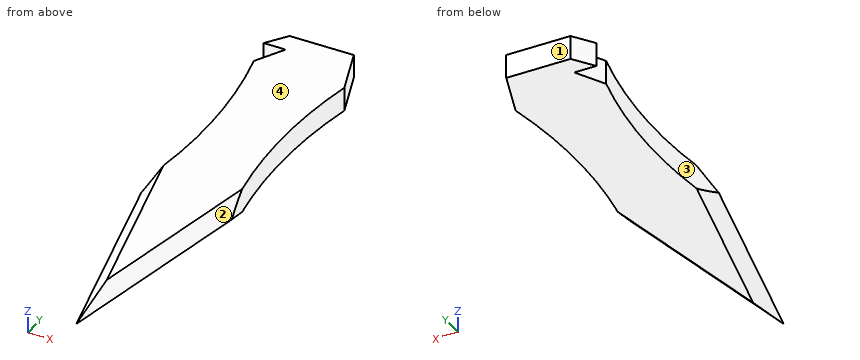
```python
from build123d import *

# Parameters (mm, degrees)
F1_DEPTH = 6.35
F3_DEPTH = 25.4
F5_DEPTH = 6.35
F6_SIZE  = 3.17499


# Not quite as in the source:
# - a fillet or chamfer is up to 0.001 mm smaller than in the source, because OpenCascade refuses the exact size


with BuildPart() as f1:
    # F0 (on Top) → F1 (new body)
    with BuildSketch(Plane.XY):
        Polygon((-21.1028610796, 36.5512275749), (-11.7370359251, 20.3291425525), (0, 29.516665265), (11.7370359251, 20.3291425525), (33.4666037048, 57.9658579735), (26.5181194991, 63.6764243245), (35.1014384706, 60.7974748498), (47.9729409095, 83.0915710438), (43.2239025831, 86.8056491017), (49.1863254635, 85.1932147405), (60.325, 104.4859649666), (44.45, 109.9852262806), (0, 63.5), (-44.45, 109.9852262806), (-60.325, 104.4859649666), (-49.1863254635, 85.1932147405), (-43.2239025831, 86.8056491017), (-47.9729409095, 83.0915710438), (-35.1014384706, 60.7974748498), (-26.5181194991, 63.6764243245), (-33.4666037048, 57.9658579735), align=None)
    extrude(amount=F1_DEPTH)

    # F2 (on face) → F3 (cut)
    with BuildSketch(Plane(origin=(0, 0, 0), x_dir=(1, 0, 0), z_dir=(0, 0, -1))):
        with BuildLine():
            ThreePointArc((-11.7370359251, -75.7744380392), (-8.6743378245, -48.0517902958), (-11.7370359251, -20.3291425525))
            Line((-11.7370359251, -20.3291425525), (-33.4666037048, -57.9658579735))
            Line((-33.4666037048, -57.9658579735), (-26.5181194991, -63.6764243245))
            Line((-26.5181194991, -63.6764243245), (-35.1014384706, -60.7974748498))
            Line((-35.1014384706, -60.7974748498), (-47.9729409095, -83.0915710438))
            Line((-47.9729409095, -83.0915710438), (-43.2239025831, -86.8056491017))
            Line((-43.2239025831, -86.8056491017), (-49.1863254635, -85.1932147405))
            Line((-49.1863254635, -85.1932147405), (-60.325, -104.4859649666))
            Line((-60.325, -104.4859649666), (-44.45, -109.9852262806))
            Line((-44.45, -109.9852262806), (-11.7370359251, -75.7744380392))
        make_face()
        with BuildLine():
            Line((33.4666037048, -57.9658579735), (11.7370359251, -20.3291425525))
            ThreePointArc((11.7370359251, -20.3291425525), (8.6743378245, -48.0517902958), (11.7370359251, -75.7744380392))
            Line((11.7370359251, -75.7744380392), (44.45, -109.9852262806))
            Line((44.45, -109.9852262806), (60.325, -104.4859649666))
            Line((60.325, -104.4859649666), (49.1863254635, -85.1932147405))
            Line((49.1863254635, -85.1932147405), (43.2239025831, -86.8056491017))
            Line((43.2239025831, -86.8056491017), (47.9729409095, -83.0915710438))
            Line((47.9729409095, -83.0915710438), (35.1014384706, -60.7974748498))
            Line((35.1014384706, -60.7974748498), (26.5181194991, -63.6764243245))
            Line((26.5181194991, -63.6764243245), (33.4666037048, -57.9658579735))
        make_face()
    extrude(amount=-F3_DEPTH, mode=Mode.SUBTRACT)

    # F4 (on face) → F5 (join)
    with BuildSketch(Plane.XY.offset(6.35)):
        Polygon((-7.4254795909, 83.2857191563), (-11.7370359251, 75.7744380392), (0, 63.5), (11.7370359251, 75.7744380392), (7.4199811484, 88.5948985815), (-9.2232923578, 88.5948985815), (-13.126935586, 83.2857191563), align=None)
        Polygon((0, 29.516665265), (-11.7370359251, 20.3291425525), (0, -33.983334735), (11.7370359251, 20.3291425525), align=None)
    extrude(amount=-F5_DEPTH)

    # F6 (size 3.175 in the source; OpenCascade refuses exactly that, so slightly less here)
    f6_edges = [f1.edges().sort_by_distance(p)[0] for p in [
        (5.868518, -6.827096, 6.35),
        (-5.868518, -6.827096, 6.35),
        (5.868518, -6.827096, 0),
        (-5.868518, -6.827096, 0),
    ]]
    chamfer(f6_edges, length=F6_SIZE)


solid = f1.part
```
Here's how the part is built. I have some questions about the finished solid (model axes, mm). Face numbers are marked on the shaded views. Coordinates: 2 decimals unless noted, no trailing zeros. Write each loop counter-clockwise with the first axis right and the second up, starting at its lowest first coordinate (ties: lowest second). Pieces come first, ordered by that corner, then holes. Notation, with made-up numbers: (68.5, -16) - (86.5, -16) arc R19 cw to (86.5, 12) - close; hole circle Ø4 at (-16.75, 34). An arc over 180 degrees is marked (long way). One line per item, written item: value.
1) We'd pull the mould along Y, two halves only. Please class the marked faces 1, 2, 3 and 4: pulls with the +Y half, pulls with the -Y half, needs draft (parallel to the pull), parting line crosses it, or undercut.
Model answer:
face 1: pulls with the +Y half
face 2: pulls with the -Y half
face 3: undercut
face 4: needs draft
2) I need wall thicknesses on line 1 along X through (y, z) = (67.5, 2.25); line 2 along X through (y, z) = (8.5, 1); line 3 along Z through (x, y) = (5, -5). Which ranges of each line are inside material? Lowest first, please.
Model answer:
line 1: x = -10.17 to 10.17
line 2: x = -6.96 to 6.96
line 3: z = 1.94 to 4.41
3) I'm going to push flat-ended pins straight in: P1, Ø3, axis at y = 40.5, z = 3, coming from the +X side; P2, Ø1.5, axis at y = 12.5, z = 3.5, coming from the +X side; P3, Ø2, axis at y = -16, z = 5.5, coming from the +X side. Where does each tip first touch, or does it pass through?
Model answer:
P1: stops at x = 9
P2: stops at x = 10.19
P3: stops at x = 2.55
4) Suppose I cut it at B-B on z = 1.5. Write out the boundary of the cut face in (x, y), and give its area (3 significant figures).
Model answer:
outline: (-13.13, 83.29) - (-7.43, 83.29) - (-11.74, 75.77) arc R127 cw to (-10.9, 24.38) - (0, -26.05) - (10.9, 24.38) arc R127 cw to (11.74, 75.77) - (7.42, 88.59) - (-9.22, 88.59) - close
area: 1,790 mm²
5) Suppose I cut it at C-C on y = 25.5. Write out the boundary of the cut face in (x, z), and give its area (3 significant figures).
Model answer:
outline: (-10.69, 1.06) - (-9.61, 0) - (9.61, 0) - (10.69, 1.06) - (10.69, 5.29) - (9.61, 6.35) - (-9.61, 6.35) - (-10.69, 5.29) - close
area: 133 mm²
